For this review, take the finished solid that the model builds, in its own axes (mm). Face numbers are marked on the shaded views. A direction names the side the tool comes from. Round coordinates to 2 decimals unless told otherwise and drop trailing zeros. Order: outer loops, then holes, each group sorted by start corner. A loop starts at its lowest first (then second) coordinate and runs counter-clockwise, first axis right, second up. Notation, with made-up numbers: M 44,-26 L 93,-26 A15 ccw 93,-16 Z; hole C 16,72.5 d3. An arc over 180 degrees is marked long. Answer as a JSON object with one key per item and string values.
from build123d import *

# Parameters (mm, degrees)
SKETCH1_R               = 18.75
BASE_EXTRUDE_DEPTH      = 45
CUT_EXTRUDE1_DEPTH      = 53.231456039
CUT_EXTRUDE1_DEPTH_BACK = 53.231456039
CUT_EXTRUDE5_DEPTH      = 53.231456197
CUT_EXTRUDE5_DEPTH_BACK = 53.231456197
CUT_EXTRUDE6_DEPTH      = 53.231456197
CUT_EXTRUDE6_DEPTH_BACK = 53.231456197
SKETCH11_R              = 4.75
SKETCH12_R              = 4.75
CUT_EXTRUDE7_DEPTH      = 53.231456197


with BuildPart() as part:
    # Sketch1 → Base-Extrude (new body)
    with BuildSketch(Plane(origin=(0, 0, 0), x_dir=(-1, 0, 0), z_dir=(0, 1, 0))):
        with Locations(Location((0, 0, 0), (0, 0, 270))):
            Circle(SKETCH1_R)
    extrude(amount=BASE_EXTRUDE_DEPTH)

    # Sketch2 → Cut-Extrude1 (cut, two sides: drawn at the far end of the back side and taken through both)
    with BuildSketch(Plane.XY.offset(-CUT_EXTRUDE1_DEPTH_BACK)):
        with BuildLine():
            Line((-18.75, -127.153745139), (-18.75, 0))
            Line((-18.75, 0), (-18.75, 30))
            ThreePointArc((-18.75, 30), (-12.357975624, 27.051515435), (-9.75, 20.513167019))
            Line((-9.75, 20.513167019), (-9.75, 9.75))
            ThreePointArc((-9.75, 9.75), (0, 0), (9.75, 9.75))
            Line((9.75, 9.75), (9.75, 20.513167019))
            ThreePointArc((9.75, 20.513167019), (12.357975624, 27.051515435), (18.75, 30))
            Line((18.75, 30), (18.75, 0))
            Line((18.75, 0), (18.75, -127.153745139))
            Line((18.75, -127.153745139), (18.75, -381.461235416))
            Line((18.75, -381.461235416), (-18.75, -381.461235416))
            Line((-18.75, -381.461235416), (-18.75, -127.153745139))
        make_face()
    extrude(amount=CUT_EXTRUDE1_DEPTH + CUT_EXTRUDE1_DEPTH_BACK, mode=Mode.SUBTRACT)

    # Sketch8 → Cut-Extrude5 (cut, two sides: drawn at the far end of the back side and taken through both)
    with BuildSketch(Plane(origin=(0, 0, 0), x_dir=(0, 0, -1), z_dir=(1, 0, 0)).offset(-CUT_EXTRUDE5_DEPTH_BACK)):
        Polygon((-10.16, -116.972671553), (-10.16, 0), (-10.16, 29.145238826), (10.16, 29.145238826), (10.16, 0), (10.16, -116.972671553), (10.16, -350.918014658), (-10.16, -350.918014658), align=None)
    extrude(amount=CUT_EXTRUDE5_DEPTH + CUT_EXTRUDE5_DEPTH_BACK, mode=Mode.SUBTRACT)

    # Sketch11 → Cut-Extrude6 (cut, two sides: drawn at the far end of the back side and taken through both)
    with BuildSketch(Plane.XY.offset(-CUT_EXTRUDE6_DEPTH_BACK)):
        with Locations(Location((0, 9.75, 0), (0, 0, 90))):
            Circle(SKETCH11_R)
    extrude(amount=CUT_EXTRUDE6_DEPTH + CUT_EXTRUDE6_DEPTH_BACK, mode=Mode.SUBTRACT)

    # Sketch12 → Cut-Extrude7 (cut, through all)
    with BuildSketch(Plane(origin=(0, 45, 0), x_dir=(-1, 0, 0), z_dir=(0, 1, 0))):
        with Locations(Location((0, 0, 0), (0, 0, 90))):
            Circle(SKETCH12_R)
    extrude(amount=-CUT_EXTRUDE7_DEPTH, mode=Mode.SUBTRACT)


solid = part.part
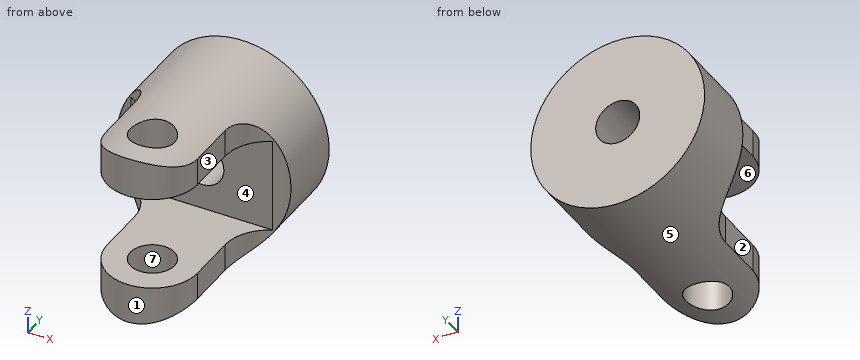
1) Add section B-B on x = 0. State the section outline as (y, z) points.
Geometry check:
{"outline": "M 0,-18.75 L 5,-18.75 L 5,-10.16 L 0,-10.16 Z; M 0,10.16 L 5,10.16 L 5,18.75 L 0,18.75 Z; M 14.5,-18.75 L 45,-18.75 L 45,-4.75 L 29.15,-4.75 L 29.15,-10.16 L 14.5,-10.16 Z; M 14.5,10.16 L 29.15,10.16 L 29.15,4.75 L 45,4.75 L 45,18.75 L 14.5,18.75 Z"}
2) Add section D-D on y = 9. State the section outline as (x, z) points, and give its area (3 significant figures).
Geometry check:
{"outline": "M -9.72,-16.03 A18.75 ccw -4.69,-18.15 L -4.69,-10.16 L -9.72,-10.16 Z; M -9.72,10.16 L -4.69,10.16 L -4.69,18.15 A18.75 ccw -9.72,16.03 Z; M 4.69,-18.15 A18.75 ccw 9.72,-16.03 L 9.72,-10.16 L 4.69,-10.16 Z; M 4.69,10.16 L 9.72,10.16 L 9.72,16.03 A18.75 ccw 4.69,18.15 Z", "area": "142 mm²"}
3) For L1, parallel to X at y = 9.75, z = -13; L2, parallel to X at y = 41, z = 0; L3, parallel to Z at x = -4, y = 18, list the stretches that pass through material, from the lowest coordinate up.
Geometry check:
{"L1": "x = -9.75 to -4.75, 4.75 to 9.75", "L2": "x = -18.75 to -4.75, 4.75 to 18.75", "L3": "z = -18.32 to -10.16, 10.16 to 18.32"}
4) Insertion check: P1, Ø3, axis at y = 15.5, z = -14.5, coming from the +X side; P2, Ø3, axis at y = 31.5, z = -5, coming from the +X side; P3, Ø2, axis at y = 31.5, z = 7.5, coming from the -X side. Each pin has a flat end and moves straight along its axis. Give the tip position at first contact, or say it passes through.
Geometry check:
{"P1": "stops at x = 9.75", "P2": "stops at x = 18.42", "P3": "stops at x = -17.59"}
5) Add section C-C on y = 26.5. State the section outline as (x, z) points, and give its area (3 significant figures).
Geometry check:
{"outline": "M -11.87,-14.51 A18.75 ccw 11.87,-14.51 L 11.87,-10.16 L -11.87,-10.16 Z; M -11.87,10.16 L 11.87,10.16 L 11.87,14.51 A18.75 ccw -11.87,14.51 Z", "area": "344 mm²"}
6) Add section A-A on z = 0. State the section outline as (x, y) points.
Geometry check:
{"outline": "M -18.75,30 A9.5 cw -15.28,29.15 L -4.75,29.15 L -4.75,45 L -18.75,45 Z; M 4.75,29.15 L 15.28,29.15 A9.5 cw 18.75,30 L 18.75,45 L 4.75,45 Z"}
7) Machinability: for the marked faces 1, 2, 3 and 4, which of the approach directions +Z, -Z, +X, -X, +Y, -Y give a long, thin tool a straight path to every point of the face, cutting with its end or side? Answer none if there is none.
Geometry check:
{"face 1": "+Z, -Z, -Y", "face 2": "+Z, -Z, -X, -Y", "face 3": "+Z, -Z, +X, -Y", "face 4": "+X, -X, -Y"}
8) Mouldability with a two-part tool opening along Z and no side actions: class the marked faces 5, 6 and 7 as +Z half, -Z half, draft (parallel to the pull), parting line (faces both ways), or undercut.
Geometry check:
{"face 5": "parting line", "face 6": "undercut", "face 7": "draft"}
